```python
from build123d import *

# Parameters (mm, degrees)
F0_W     = 100
F0_H     = 20
F1_DEPTH = 50
F2_R     = 5
F3_T     = -2.5


# Not quite as in the source:
# - a shell that OpenCascade refuses in one call is made with other operations: the cavity is built on its own and cut out


with BuildPart() as f1:
    # F0 (on Right) → F1 (new body)
    with BuildSketch(Plane.YZ):
        Rectangle(F0_W, F0_H)
    extrude(amount=F1_DEPTH)

    # F2
    f2_edges = [f1.edges().sort_by_distance(p)[0] for p in [
        (25, -50, -10),
        (50, -50, 0),
        (0, -50, 0),
        (0, 0, -10),
        (50, 0, -10),
        (50, 50, 0),
        (0, 50, 0),
        (25, 50, -10),
        (25, 50, 10),
        (0, 0, 10),
        (25, -50, 10),
        (50, 0, 10),
    ]]
    fillet(f2_edges, radius=F2_R)

    # F3: a shell. OpenCascade refuses it in one call, so the cavity is built on its own and cut out:
    # the body offset inwards by the wall thickness, plus a prism from it out through each open face.
    f3_core = offset(f1.part, amount=F3_T, mode=Mode.PRIVATE)
    f3_exits = [f3_core.faces().sort_by_distance(p)[0] for p in [
        (25, 0, 7.5),
    ]]
    add(f3_core, mode=Mode.SUBTRACT)
    extrude(f3_exits, amount=-F3_T, mode=Mode.SUBTRACT)


solid = f1.part
```
Geometry: final body of the model. Coordinates: model frame, mm. A direction names the side the tool comes from. Round coordinates to 2 decimals unless told otherwise and drop trailing zeros. Write each loop counter-clockwise with the first axis right and the second up, starting at its lowest first coordinate (ties: lowest second). Pieces come first, ordered by that corner, then holes. Notation, with made-up numbers: M 3,-38 L 60,-38 A23 ccw 60,-1 Z; hole C 67.25,9 d5. An arc over 180 degrees is marked long. Answer in a Markdown table with one row per item. Add a question column.
(1) Cut plane D-D, the plane z = 8.5. Return the cut outline in (x, y).
(2) Ray query, L1, parallel to Y at x = 13, z = -0.75; L2, parallel to X at y = -5, z = 2.25; L3, parallel to Y at x = 46, z = 5.5. Return the intervals inside material, ascending.
(3) Cut plane C-C, the plane x = 11. Return the cut outline in (y, z), then the cut area to 3 significant figures.
(4) Contact query for flat-ended pins moving along their axis: pin 1 (1.5 mm diameter, centred on x = 16.5, y = -1.5, fed in from +Z); pin 2 (2 mm diameter, centred on x = 27.5, z = 9, fed in from -Y); pin 3 (0.8 mm diameter, centred on x = 29, z = 9, fed in from +Y). Output: stop coordinate, or through.
(5) Cut plane B-B, the plane y = -27.5. Return the cut outline in (x, z), then the cut area to 3 significant figures.
(6) Reachability of faces 4 (the face through (5, -1, 9)), 5 (the face through (25.28, 46.748, -6.787)), 6 (the face through (2, 1, 9)) from +Z, -Z, +X, -X, +Y, -Y: full face, straight path, thin tool, end or side. Return the list, or none.
(7) Cut plane A-A, the plane z = 3.25. Return the cut outline in (x, y).
(8) Draft query along Y for faces 1 (the face through (3.252, 46.787, 0.07)), 2 (the face through (25, 49, 8)), 3 (the face through (25, -50, 0)). Return one class per face: pulls with the +Y half, pulls with the -Y half, needs draft (parallel to the pull), parting line crosses it, or undercut.
Established:
| question | item | result |
|---|---|---|
| 1 | outline | M 1.43,-45 A3.57 ccw 5,-48.57 L 45,-48.57 A3.57 ccw 48.57,-45 L 48.57,45 A3.57 ccw 45,48.57 L 5,48.57 A3.57 ccw 1.43,45 Z; hole M 5,-45 L 45,-45 L 45,45 L 5,45 Z |
| 2 | L1 | -50 to -47.5, 47.5 to 50 |
| 2 | L2 | 0 to 2.5, 47.5 to 50 |
| 2 | L3 | -49.87 to -47.24, 47.24 to 49.87 |
| 3 | outline | M -50,-5 A5 ccw -45,-10 L 45,-10 A5 ccw 50,-5 L 50,5 A5 ccw 45,10 L 45,7.5 A2.5 cw 47.5,5 L 47.5,-5 A2.5 cw 45,-7.5 L -45,-7.5 A2.5 cw -47.5,-5 L -47.5,5 A2.5 cw -45,7.5 L -45,10 A5 ccw -50,5 Z |
| 3 | area | 334 mm² |
| 4 | pin 1 | z = -7.5 |
| 4 | pin 2 | y = -49 |
| 4 | pin 3 | y = 48.47 |
| 5 | outline | M 0,-5 A5 ccw 5,-10 L 45,-10 A5 ccw 50,-5 L 50,5 A5 ccw 45,10 L 45,7.5 A2.5 cw 47.5,5 L 47.5,-5 A2.5 cw 45,-7.5 L 5,-7.5 A2.5 cw 2.5,-5 L 2.5,5 A2.5 cw 5,7.5 L 5,10 A5 ccw 0,5 Z |
| 5 | area | 209 mm² |
| 6 | face 4 | +Z |
| 6 | face 5 | none |
| 6 | face 6 | +Z, -X, +Y, -Y |
| 7 | outline | M 0,-45 A5 ccw 5,-50 L 45,-50 A5 ccw 50,-45 L 50,45 A5 ccw 45,50 L 5,50 A5 ccw 0,45 Z; hole M 2.5,-45 A2.5 ccw 5,-47.5 L 45,-47.5 A2.5 ccw 47.5,-45 L 47.5,45 A2.5 ccw 45,47.5 L 5,47.5 A2.5 ccw 2.5,45 Z |
| 8 | face 1 | undercut |
| 8 | face 2 | pulls with the +Y half |
| 8 | face 3 | pulls with the -Y half |
